Autodesk Inventor part; units mm, degrees
ref_plane "YZ Plane" through (0, 0, 0) normal (1, 0, 0) x (0, 1, 0)
ref_plane "XZ Plane" through (0, 0, 0) normal (0, 1, 0) x (-1, 0, 0)
ref_plane "XY Plane" through (0, 0, 0) normal (0, 0, 1) x (1, 0, 0)
sketch "Sketch1" plane through (0, 0, 0) normal (0, 1, 0) x (-1, 0, 0)
  line L0 (-4, 17.5) -> (-4, -17.5)
  line L1 (-4, -17.5) -> (4, -17.5)
  line L2 (4, -17.5) -> (4, 17.5)
  line L3 (4, 17.5) -> (-4, 17.5)
  line L4 (-4, 17.5) -> (4, -17.5) construction
  line L5 (-4, -17.5) -> (4, 17.5) construction
  line L6 (0, 0) -> (0, 8.89)
  line L7 (0, 0) -> (0, 12)
  circle A0 centre (0, 12) radius 1.45
  line L8 (0, 0) -> (0, -12)
  circle A1 centre (0, -12) radius 1.45
  dimension "d0" = 35
  dimension "d1" = 8
  dimension "d3" = 12
  dimension "d4" = 2.9
  dimension "d5" = 12
  dimension "d6" = 2.9
extrude "Extrusion1" add sketch "Sketch1" along normal blind 5
sketch "Sketch2" plane through (0, 5, 0) normal (0, 1, 0) x (1, 0, 0)
  line L0 (1.5, -17.5) -> (1.5, 17.5)
  line L1 (1.5, 17.5) -> (-1.5, 17.5)
  line L2 (-1.5, 17.5) -> (-1.5, -17.5)
  line L3 (-1.5, -17.5) -> (1.5, -17.5)
  line L4 (1.5, -17.5) -> (-1.5, 17.5) construction
  line L5 (1.5, 17.5) -> (-1.5, -17.5) construction
  point P0 (0, 0)
  dimension "d9" = 35
  dimension "d10" = 3
extrude "Extrusion2" add sketch "Sketch2" along normal blind 18
sketch "Sketch3" plane through (1.5, 5, 17.5) normal (1, 0, 0) x (0, 0, -1)
  line L0 (0, 18) -> (35, 18)
  line L1 (17.5, 18) -> (17.5, 9)
  line L2 (17.5, 18) -> (26.5, 18) construction
  line L3 (17.5, 9) -> (8.61, 9)
  line L4 (17.5, 9) -> (26.39, 9)
  line L5 (17.5, 9) -> (26.39, 9) construction
  circle A0 centre (8.61, 9) radius 6.35
  circle A1 centre (26.39, 9) radius 6.35
  point P0 (17.5, -5)
  dimension "d13" = 9
  dimension "d14" = 90
  dimension "d15" = 8.89
  dimension "d16" = 90
  dimension "d17" = 8.89
  dimension "d18" = 0
  dimension "d19" = 12.7
  dimension "d20" = 12.7
extrude "Extrusion3" cut sketch "Sketch3" against normal blind 15
fillet "Fillet1" radius 2 2 edges at (0, 23, -17.5) (0, 23, 17.5)
fillet "Fillet2" radius 1 4 edges at (4, 2.5, -17.5) (-4, 2.5, -17.5) (4, 2.5, 17.5) (-4, 2.5, 17.5)
fillet "Fillet3" radius 0.75 10 edges at (1.5, 22.4142, -16.9142) (1.5, 13, -17.5) (1.5, 22.4142, 16.9142) (1.5, 13, 17.5) (1.5, 23, 0) (-1.5, 22.4142, 16.9142) (-1.5, 13, 17.5) (-1.5, 22.4142, -16.9142) (-1.5, 13, -17.5) (-1.5, 23, 0)
fillet "Fillet4" radius 0.75 10 edges at (3.7071, 5, -17.2071) (-2.25, 5, -17.5) (2.25, 5, -17.5) (-3.7071, 5, -17.2071) (-4, 5, 0) (-3.7071, 5, 17.2071) (-2.25, 5, 17.5) (2.25, 5, 17.5) (3.7071, 5, 17.2071) (4, 5, 0)
properties part number "Sonar Mount" material "ABS Plastic"
Verification items for the finished model (mm, model axes). A direction names the side the tool comes from. Round coordinates to 2 decimals unless told otherwise and drop trailing zeros. Loops run counter-clockwise (first coordinate to the right, second up) from the corner with the lowest first, then second, coordinate; pieces in that order, holes last. Notation, with made-up numbers: (-20.5, 73) - (30.5, 73) arc R38 ccw to (30.5, 111) - close; hole circle Ø6 at (9, 70.25). An arc over 180 degrees is marked (long way). Answer in a Markdown table with one row per item. Add a question column.
Q1. Section check A-A on z = -8.89. Enter the section's corners in (x, y), plus the area to 3 significant figures.
Q2. Release check for a two-part mould opening along X. For faces 1 (the face through (4, 2, 0)), 2 (the face through (0, 5, 12)), 3 (the face through (0, 5, -12)), 4 (the face through (-1.5, 14, 0)) record: pulls with the +X half, pulls with the -X half, needs draft (parallel to the pull), parting line crosses it, or undercut.
Q3. Gauge pin test, flat ends, axial feed: pin 1 (1.4 mm diameter, centred on x = -0.5, z = 11.5, fed in from -Y); pin 2 (11.5 mm diameter, centred on y = 14, z = 8.89, fed in from +X); pin 3 (5 mm diameter, centred on y = 19.5, z = -3.5, fed in from +X); pin 4 (1.4 mm diameter, centred on x = -2, z = -3.5, fed in from +Y). Record the tip position at first contact, or that the pin passes through.
Q4. Section check D-D on x = 2.5. Enter the section's corners in (y, z), plus the area to 3 significant figures.
Q5. Section check B-B on x = 0. Enter the section's corners in (y, z), plus the area to 3 significant figures.
Q6. Material ranges on line 1 (Z direction, x = 0, y = 1.5); line 2 (X direction, y = 7.25, z = -15); line 3 (Z direction, x = -0.5, y = 13), recorded low to high.
Q7. Tool access check on faces 5 (the face through (0, 8, -17.5)), 6 (the face through (0.314, 2.465, -10.584)), 7 (the face through (-2, 5, 0)), 8 (the face through (0, 8, 17.5)), 9 (the face through (2, 5, 0)). Record the directions out of +Z, -Z, +X, -X, +Y, -Y that give a thin tool (end or side, any length) a straight path to the whole face; none if there is none.
Q8. Section check C-C on y = 14.5. Enter the section's corners in (x, z).
Found:
| question | item | result |
|---|---|---|
| 1 | outline | (-4, 0) - (4, 0) - (4, 4.25) arc R0.75 ccw to (3.25, 5) - (1.5, 5) - (1.5, 7.65) - (-1.5, 7.65) - (-1.5, 5) - (-3.25, 5) arc R0.75 ccw to (-4, 4.25) - close; (-1.5, 20.35) - (1.5, 20.35) - (1.5, 22.25) arc R0.75 ccw to (0.75, 23) - (-0.75, 23) arc R0.75 ccw to (-1.5, 22.25) - close |
| 1 | area | 55.4 mm² |
| 2 | face 1 | pulls with the +X half |
| 2 | face 2 | undercut |
| 2 | face 3 | undercut |
| 2 | face 4 | pulls with the -X half |
| 3 | pin 1 | stops at y = 5 |
| 3 | pin 2 | passes through |
| 3 | pin 3 | stops at x = 1.5 |
| 3 | pin 4 | stops at y = 22.76 |
| 4 | outline | (0, -17.5) - (4.25, -17.5) arc R0.75 ccw to (5, -16.75) - (5, 16.75) arc R0.75 ccw to (4.25, 17.5) - (0, 17.5) - close |
| 4 | area | 175 mm² |
| 5 | outline | (0, -17.5) - (21, -17.5) arc R2 ccw to (23, -15.5) - (23, 15.5) arc R2 ccw to (21, 17.5) - (0, 17.5) - (0, 13.45) - (5, 13.45) - (5, 10.55) - (0, 10.55) - (0, -10.55) - (5, -10.55) - (5, -13.45) - (0, -13.45) - close; hole circle Ø12.7 at (14, -8.89); hole circle Ø12.7 at (14, 8.89) |
| 5 | area | 521 mm² |
| 6 | line 1 | z = -17.5 to -13.45, -10.55 to 10.55, 13.45 to 17.5 |
| 6 | line 2 | x = -1.5 to 1.5 |
| 6 | line 3 | z = -17.5 to -15.16, -2.62 to 2.62, 15.16 to 17.5 |
| 7 | face 5 | -Z, +X, -X, +Y, -Y |
| 7 | face 6 | -Y |
| 7 | face 7 | +Z, -Z, -X, +Y |
| 7 | face 8 | +Z, +X, -X, +Y, -Y |
| 7 | face 9 | +Z, -Z, +X, +Y |
| 8 | outline | (-1.5, -16.75) arc R0.75 ccw to (-0.75, -17.5) - (0.75, -17.5) arc R0.75 ccw to (1.5, -16.75) - (1.5, -15.22) - (-1.5, -15.22) - close; (-1.5, -2.56) - (1.5, -2.56) - (1.5, 2.56) - (-1.5, 2.56) - close; (-1.5, 15.22) - (1.5, 15.22) - (1.5, 16.75) arc R0.75 ccw to (0.75, 17.5) - (-0.75, 17.5) arc R0.75 ccw to (-1.5, 16.75) - close |
